Autodesk Inventor part; units mm, degrees
ref_plane "Work Plane2" through (2.032, 0, 0) normal (0, 1, 0) x (1, 0, 0)
ref_plane "YZ Plane" through (0, 0, 0) normal (1, 0, 0) x (0, 1, 0)
ref_plane "XZ Plane" through (0, 0, 0) normal (0, 1, 0) x (-1, 0, 0)
sketch "Sketch1" plane through (0, 0, 0) normal (0, 0, 1) x (1, 0, 0)
  line L0 (4.3434, 0) -> (19.05, 0)
  line L1 (19.05, 0) -> (19.05, 3.175)
  line L2 (19.05, 3.175) -> (3.8862, 3.175)
  line L3 (0.935, 5.7404) -> (0, 5.7404)
  line L4 (-3.81, 0) -> (22.86, 0)
  line L5 (0, -1.1481) -> (0, 6.8885)
  line L6 (0, 3.5941) -> (3.3098, 1.9439)
  line L7 (3.3098, 1.9439) -> (4.3434, 0)
  line L8 (3.8862, 3.175) -> (0.935, 5.7404)
  line L9 (0, 5.7404) -> (0, 3.5941)
  dimension "d2" = 6.35
  dimension "d3" = 11.4808
  dimension "d4" = 4.3434
  dimension "d5" = 7.1882
  dimension "d6" = 26.5
  dimension "d7" = 62
  dimension "d13" = 41
  dimension "d14" = 3.8862
  dimension "d15" = 19.05
revolve "Body" add sketch "Sketch1" angle 360 about axis through (4.3434, 0, 0) along (1, 0, 0) contours L7 L6 L5 L3 L8 L2 L1 L0
sketch "Sketch2" plane through (0, 0, 0) normal (-1, 0, 0) x (0, 0, 1)
  line L0 (0, -8.0366) -> (0, 8.0366)
  line L1 (-8.0366, 0) -> (8.0366, 0)
  line L2 (0, 3.5941) -> (0, 0) construction
  line L3 (0, 0) -> (3.5941, 0) construction
  arc A0 (1.198, 0) -> (0, 1.198) centre (0, 0) ccw
  line L4 (0, 0) -> (0.7947, 0.7947) construction
  arc A1 (1.797, 0) -> (0, 1.797) centre (0, 0) ccw construction
  line L5 (0.4572, 3.5649) -> (0.4751, 1.7331)
  line L6 (3.5649, 0.4572) -> (1.7331, 0.4751)
  arc A2 (0.4751, 1.7331) -> (1.7331, 0.4751) centre (1.7455, 1.7455) ccw
  arc A3 (3.5941, 0) -> (3.5649, 0.4572) centre (0, 0) ccw
  arc A4 (0.4572, 3.5649) -> (0, 3.5941) centre (0, 0) ccw
  arc A5 (3.5649, 0.4572) -> (0.4572, 3.5649) centre (0, 0) ccw
  line L7 (0.4572, -3.5649) -> (0.4751, -1.7331)
  line L8 (3.5649, -0.4572) -> (1.7331, -0.4751)
  arc A6 (1.7331, -0.4751) -> (0.4751, -1.7331) centre (1.7455, -1.7455) ccw
  arc A7 (3.5649, -0.4572) -> (3.5941, 0) centre (0, 0) ccw
  arc A8 (0, -3.5941) -> (0.4572, -3.5649) centre (0, 0) ccw
  arc A9 (0.4572, -3.5649) -> (3.5649, -0.4572) centre (0, 0) ccw
  line L9 (-0.4572, 3.5649) -> (-0.4751, 1.7331)
  line L10 (-3.5649, 0.4572) -> (-1.7331, 0.4751)
  arc A10 (-1.7331, 0.4751) -> (-0.4751, 1.7331) centre (-1.7455, 1.7455) ccw
  arc A11 (-3.5649, 0.4572) -> (-3.5941, 0) centre (0, 0) ccw
  arc A12 (0, 3.5941) -> (-0.4572, 3.5649) centre (0, 0) ccw
  arc A13 (-0.4572, 3.5649) -> (-3.5649, 0.4572) centre (0, 0) ccw
  arc A14 (-3.5649, -0.4572) -> (-0.4572, -3.5649) centre (0, 0) ccw
  arc A15 (-0.4572, -3.5649) -> (0, -3.5941) centre (0, 0) ccw
  arc A16 (-3.5941, 0) -> (-3.5649, -0.4572) centre (0, 0) ccw
  line L11 (-3.5649, -0.4572) -> (-1.7331, -0.4751)
  arc A17 (-0.4751, -1.7331) -> (-1.7331, -0.4751) centre (-1.7455, -1.7455) ccw
  line L12 (-0.4572, -3.5649) -> (-0.4751, -1.7331)
  dimension "d18" = 45
  dimension "d19" = 2.3961
  dimension "d20" = 3.5941
  dimension "d21" = 7.1882
  dimension "d22" = 0.4572
extrude "Slot" add sketch "Sketch2" against normal up to next contours A2 L5 A5 L6 | L9 A10 L10 A13 | L7 A6 L8 A9 | A14 L11 A17 L12
fillet "Fillet1" radius 0.1829 4 edges at (0, 3.5941, 0) (0, 0, 3.5941) (0, -3.5941, 0) (0, 0, -3.5941)
thread "Thread"
chamfer "Chamfer1" distance 0.9525 distance2 0.9525 1 edges at (19.05, -3.175, 0) measured on face at (19.05, -0.3658, -0.0841)
ref_plane "Work Plane2" through (2.032, 0, 0) normal (0, 1, 0) x (1, 0, 0)
equation "\"d2\" = GD"
equation "\"d3\" = KOD"
equation "\"d4\" = INTI"
equation "\"d5\" = SDM"
equation "\"d13\" = 0.5 * SEWI"
equation "\"d14\" = KOH"
equation "\"d15\" = NLG"
equation "\"d19\" = 0.333333 * SDM"
equation "\"d20\" = 0.5 * SDM"
equation "\"d21\" = SDM"
equation "\"d22\" = 0.5 * SBR"
equation "\"d45\" = INTI"
equation "\"d25\" = 0.2 * SBR"
equation "\"d9\" = GEL"
equation "\"d11\" = -0.5 * SPD + 0.5 * GD"
equation "\"d12\" = GUL"
equation "\"GD\" = NND"
equation "\"NLG\" = 19.05"
equation "\"GEL\" = 11.9888"
equation "\"KOD\" = 11.4808"
equation "\"KOH\" = 3.8862"
equation "\"SDM\" = 7.1882"
equation "\"INTI\" = 4.3434"
equation "\"SBR\" = 0.9144"
equation "\"GUL\" = 0.75 * GAL"
equation "\"SPD\" = 4.445"
equation "\"SEWI\" = 82deg"
equation "\"d0\" = NLG"
equation "\"d1\" = KOH"
equation "\"d17\" = SDM"
equation "\"TOA\" = 30deg"
equation "\"THREADDIA\" = 6.35"
equation "\"BDM\" = NND"
equation "\"NND\" = 6.35"
equation "\"GAL\" = 1.27"
equation "\"GD1\" = SPD"
properties part number "ANSI B18.6.3 - 1/4-20 x 3/4, CRFCHMSTII(5)" material "Steel, Mild"
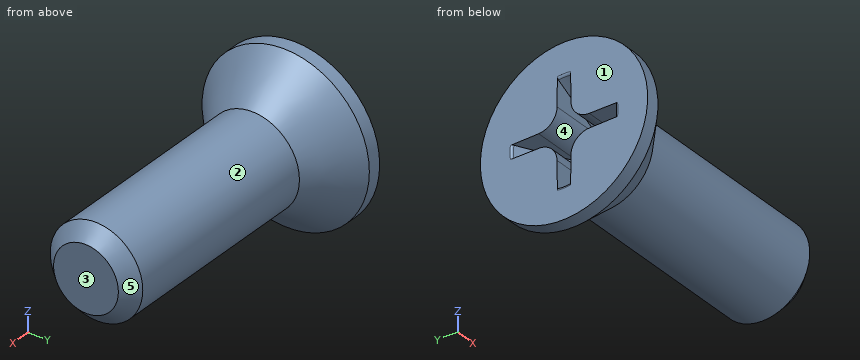
Geometry check sheet. Reference: the model listing, model coordinates, mm. Face numbers are marked on the shaded views. A direction names the side the tool comes from. Give positions to 0.01 mm unless a question says otherwise; leave off trailing zeros. Order: outer loops, then holes, each group sorted by start corner. A loop starts at its lowest first (then second) coordinate and runs counter-clockwise, first axis right, second up. Notation, with made-up numbers: (2.5, 19.5) - (25.5, 19.5) arc R9 ccw to (25.5, 28.5) - close; hole circle Ø11 at (14, 13). An arc over 180 degrees is marked (long way). Answer as a JSON object with one key per item and string values.
(1) Cross-section at A-A (x = 14.75). Record the cut outline in (y, z) (3 decimals).
Report:
{"outline": "circle Ø6.35 at (0, 0)"}
(2) Tool access check on the marked faces 1 and 2. Record the directions out of +Z, -Z, +X, -X, +Y, -Y that give a thin tool (end or side, any length) a straight path to the whole face; none if there is none.
Report:
{"face 1": "+Z, -Z, -X, +Y, -Y", "face 2": "+X"}
(3) Material ranges on line 1 (X direction, y = 3, z = -2); line 2 (X direction, y = 1.5, z = 0); line 3 (Z direction, x = 1.75, y = 2), recorded low to high.
Report:
{"line 1": "0 to 3.39", "line 2": "3.55 to 19.05", "line 3": "-4.62 to -0.47, 0.47 to 4.62"}
(4) Draft check along Y on the marked faces 3, 4 and 5. Enter one of: released by +Y, released by -Y, zero draft, split by the parting line, or undercut.
Report:
{"face 3": "zero draft", "face 4": "undercut", "face 5": "split by the parting line"}
(5) Depth check by flat-ended pin: pin 1 Ø3 at (x, y) = (16, 1) entering from +Z (3 decimals); pin 2 Ø6 at (x, z) = (3.5, -2.5) entering from +Y; pin 3 Ø4 at (x, y) = (15, -4) entering from -Z. Enter the tip coordinate at first touch or a pass-through.
Report:
{"pin 1": "z = 3.175", "pin 2": "y = 5.66", "pin 3": "z = -2.47"}
